```python
from build123d import *
from build123d.topology import SkipClean

# Parameters (mm, degrees)
SKETCH1_R             = 8
BOSS_EXTRUDE1_DEPTH   = 47.5
BOSS_EXTRUDE2_START   = 10
BOSS_EXTRUDE2_DEPTH   = 10
SKETCH3_R             = 9
BOSS_EXTRUDE3_DEPTH   = 4
LPATTERN1_COUNT       = 6
LPATTERN1_PITCH       = 95
BODY_MOVE_COPY1_ANGLE = 60
BODY_MOVE_COPY2_ANGLE = 120
BODY_MOVE_COPY3_ANGLE = 60
BODY_MOVE_COPY4_ANGLE = 120
BODY_MOVE_COPY5_ANGLE = 180
SKETCH4_R             = 8
BOSS_EXTRUDE4_DEPTH   = 10
SKETCH5_R             = 9
BOSS_EXTRUDE5_DEPTH   = 5
SKETCH6_R             = 7.5
BOSS_EXTRUDE6_DEPTH   = 5
SKETCH7_R             = 8
BOSS_EXTRUDE7_DEPTH   = 7.5
SKETCH8_R             = 9
BOSS_EXTRUDE8_DEPTH   = 5
SKETCH9_R             = 7.5
BOSS_EXTRUDE9_DEPTH   = 38
SKETCH10_R            = 25
SKETCH10_R_2          = 2.5
BOSS_EXTRUDE10_DEPTH  = 10
SKETCH11_R            = 2.5
CUT_EXTRUDE1_DEPTH    = 15
FILLET1_R             = 2


with BuildPart() as part:
    # Sketch1 → Boss-Extrude1 (new, symmetric)
    with BuildSketch(Plane(origin=(0, 0, 0), x_dir=(0, 0, -1), z_dir=(1, 0, 0))):
        Circle(SKETCH1_R)
    extrude(amount=BOSS_EXTRUDE1_DEPTH, both=True)

    # Sketch2 → Boss-Extrude2 (add)
    with BuildSketch(Plane(origin=(0, 0, 0), x_dir=(0, 0, -1), z_dir=(1, 0, 0)).offset(BOSS_EXTRUDE2_START)):
        with BuildLine():
            Line((-8.746197071, -4.848096202), (-3.807936598, -13.756953924))
            ThreePointArc((-3.807936598, -13.756953924), (0, -16), (3.807936598, -13.756953924))
            Line((3.807936598, -13.756953924), (8.746197071, -4.848096202))
            ThreePointArc((8.746197071, -4.848096202), (0, 10), (-8.746197071, -4.848096202))
        make_face()
    boss_extrude2 = extrude(amount=BOSS_EXTRUDE2_DEPTH)

    # Mirror1: Boss-Extrude2 across plane
    add(boss_extrude2.mirror(Plane(origin=(0, 0, 0), x_dir=(0, 0, 1), z_dir=(1, 0, 0))))

    # Sketch3 → Boss-Extrude3 (add, symmetric)
    with BuildSketch(Plane(origin=(0, 0, 0), x_dir=(0, 0, -1), z_dir=(1, 0, 0))):
        Circle(SKETCH3_R)
    extrude(amount=BOSS_EXTRUDE3_DEPTH, both=True)


with BuildPart() as lpattern1_1:
    # LPattern1: pattern copy
    add(part.part.moved(Location(Vector(-1, 0, 0) * (1 * LPATTERN1_PITCH))))


with BuildPart() as lpattern1_2:
    # LPattern1: pattern copy
    add(part.part.moved(Location(Vector(-1, 0, 0) * (2 * LPATTERN1_PITCH))))


with BuildPart() as lpattern1_3:
    # LPattern1: pattern copy
    add(part.part.moved(Location(Vector(-1, 0, 0) * (3 * LPATTERN1_PITCH))))


with BuildPart() as lpattern1_4:
    # LPattern1: pattern copy
    add(part.part.moved(Location(Vector(-1, 0, 0) * (4 * LPATTERN1_PITCH))))


with BuildPart() as lpattern1_5:
    # LPattern1: pattern copy
    add(part.part.moved(Location(Vector(-1, 0, 0) * (5 * LPATTERN1_PITCH))))


with BuildPart() as lpattern1_3_1:
    # Body-Move_Copy1: moved
    add(lpattern1_3.part.rotate(Axis((0, 0, 0), (-1, 0, 0)), BODY_MOVE_COPY1_ANGLE))


with BuildPart() as lpattern1_1_1:
    # Body-Move_Copy2: moved
    add(lpattern1_1.part.rotate(Axis((0, 0, 0), (-1, 0, 0)), BODY_MOVE_COPY2_ANGLE))


with BuildPart() as lpattern1_4_1:
    # Body-Move_Copy3: moved
    add(lpattern1_4.part.rotate(Axis((0, 0, 0), (1, 0, 0)), BODY_MOVE_COPY3_ANGLE))


with BuildPart() as lpattern1_2_1:
    # Body-Move_Copy4: moved
    add(lpattern1_2.part.rotate(Axis((0, 0, 0), (1, 0, 0)), BODY_MOVE_COPY4_ANGLE))


with BuildPart() as lpattern1_5_1:
    # Body-Move_Copy5: moved
    add(lpattern1_5.part.rotate(Axis((0, 0, 0), (1, 0, 0)), BODY_MOVE_COPY5_ANGLE))

    # Sketch4 → Boss-Extrude4 (add)
    with BuildSketch(Plane.ZY.offset(522.5)):
        Circle(SKETCH4_R)
    extrude(amount=BOSS_EXTRUDE4_DEPTH)

    # Sketch5 → Boss-Extrude5 (add)
    with BuildSketch(Plane.ZY.offset(532.5)):
        Circle(SKETCH5_R)
    extrude(amount=BOSS_EXTRUDE5_DEPTH)


with BuildPart() as lpattern1_4_2:
    add(lpattern1_4_1.part)

    # Combine1: union LPattern1_1, LPattern1_3, LPattern1_2, part, LPattern1_5
    add(lpattern1_1_1.part)
    add(lpattern1_3_1.part)
    add(lpattern1_2_1.part)
    add(part.part)
    add(lpattern1_5_1.part)

    # Sketch6 → Boss-Extrude6 (add)
    with BuildSketch(Plane.ZY.offset(537.5)):
        Circle(SKETCH6_R)
    extrude(amount=BOSS_EXTRUDE6_DEPTH)

    # Sketch7 → Boss-Extrude7 (add)
    with SkipClean():  # the faces are left unmerged after this step: merging them gives an invalid solid
        with BuildSketch(Plane(origin=(47.5, 0, 0), x_dir=(0, 0, -1), z_dir=(1, 0, 0))):
            with Locations(Location((0, 0, 0), (0, 0, 60))):
                Circle(SKETCH7_R)
        extrude(amount=BOSS_EXTRUDE7_DEPTH)
    add(lpattern1_4_2.part.scale(1), mode=Mode.REPLACE)  # the faces are merged on a copy

    # Sketch8 → Boss-Extrude8 (add)
    with SkipClean():  # the faces are left unmerged after this step: merging them gives an invalid solid
        with BuildSketch(Plane(origin=(55, 0, 0), x_dir=(0, 0, -1), z_dir=(1, 0, 0))):
            with Locations(Location((0, 0, 0), (0, 0, 60))):
                Circle(SKETCH8_R)
        extrude(amount=BOSS_EXTRUDE8_DEPTH)

    # Sketch9 → Boss-Extrude9 (add)
    with SkipClean():  # the faces are left unmerged after this step: merging them gives an invalid solid
        with BuildSketch(Plane(origin=(60, 0, 0), x_dir=(0, 0, -1), z_dir=(1, 0, 0))):
            with Locations(Location((0, 0, 0), (0, 0, 180))):
                Circle(SKETCH9_R)
        extrude(amount=BOSS_EXTRUDE9_DEPTH)

    # Sketch10 → Boss-Extrude10 (add)
    with SkipClean():  # the faces are left unmerged after this step: merging them gives an invalid solid
        with BuildSketch(Plane(origin=(98, 0, 0), x_dir=(0, 0, -1), z_dir=(1, 0, 0))):
            Circle(SKETCH10_R)
            Circle(SKETCH10_R_2, mode=Mode.SUBTRACT)
        extrude(amount=BOSS_EXTRUDE10_DEPTH)

    # Sketch11 → Cut-Extrude1 (cut)
    with SkipClean():  # the faces are left unmerged after this step: merging them gives an invalid solid
        with BuildSketch(Plane(origin=(108, 0, 0), x_dir=(0, 0, -1), z_dir=(1, 0, 0))):
            with Locations((0, 15)):
                Circle(SKETCH11_R)
            Circle(SKETCH11_R)
            with Locations((14.265847744, 4.635254916)):
                Circle(SKETCH11_R)
            with Locations((8.816778784, -12.135254916)):
                Circle(SKETCH11_R)
            with Locations((-8.816778784, -12.135254916)):
                Circle(SKETCH11_R)
            with Locations((-14.265847744, 4.635254916)):
                Circle(SKETCH11_R)
        extrude(amount=-CUT_EXTRUDE1_DEPTH, mode=Mode.SUBTRACT)

    # Fillet1
    fillet1_edges = [lpattern1_4_2.edges().sort_by_distance(p)[0] for p in [
        (98, 0, -7.5),
        (98, 0, 25),
    ]]
    fillet(fillet1_edges, radius=FILLET1_R)


solid = lpattern1_4_2.part
```
Geometry check sheet. Reference: the model listing, model coordinates, mm. A direction names the side the tool comes from. Round coordinates to 2 decimals unless told otherwise and drop trailing zeros. Order: outer loops, then holes, each group sorted by start corner. A loop starts at its lowest first (then second) coordinate and runs counter-clockwise, first axis right, second up. Notation, with made-up numbers: M -11.5,-38.5 L 42.5,-38.5 A24 ccw 42.5,-13.5 Z; hole C 45.5,-25.75 d4. An arc over 180 degrees is marked long. Answer as CSV lines item,"result".
1) Sectioned sample at A-A on x = -339. Record the cut outline in (y, z).
Entries:
outline,"C 0,0 d16"
2) Mould release check, pull along X, two halves, no side actions. Record for faces 3 (the face through (-542.5, 0, 0)), 4 (the face through (108, -5, 0)), 5 (the face through (-305, -2, 8)): +X half, -X half, draft (parallel to the pull), parting line (faces both ways), or undercut.
Entries:
face 3,"-X half"
face 4,"+X half"
face 5,"undercut"
3) Thickness scan on probe 1 along X at (y, z) = (-12.5, 4); probe 2 along X at (y, z) = (13, -2.5); probe 3 along Y at (x, z) = (-122.5, -5) (3 decimals). Record the ranges inside material, lowest first. Write a range as [from, to].
Entries:
probe 1,"[-20, -10], [10, 20], [98, 108]"
probe 2,"[-495, -485], [-465, -455], [98, 108]"
probe 3,"[-6.245, 6.245]"
4) Gauge pin test, flat ends, axial feed: pin 1 Ø14.5 at (y, z) = (-1, 0) entering from +X; pin 2 Ø4.5 at (y, z) = (4.64, 14.27) entering from -X; pin 3 Ø6 at (x, y) = (27.5, -12.5) entering from +Z; pin 4 Ø10 at (x, z) = (-88, -11.5) entering from -Y. Record the tip position at first contact, or that the pin passes through.
Entries:
pin 1,"x = 108"
pin 2,"x = -115"
pin 3,"through"
pin 4,"y = -6.61"
5) Tool access check on faces 1 (the face through (-537.5, 7.4, -2)), 2 (the face through (-175.07, -4.75, 8.8)). Record the directions out of +Z, -Z, +X, -X, +Y, -Y that give a thin tool (end or side, any length) a straight path to the whole face; none if there is none.
Entries:
face 1,"-X"
face 2,"none"
